```python
from build123d import *

# Parameters (mm, degrees)
F1_DEPTH = 8
F2_R     = 2.5
F3_R     = 5
F4_DEPTH = 5
F5_R     = 5
F6_DEPTH = 5


# Not quite as in the source:
# - a feature names something its author has since deleted; it is built from what else it names


with BuildPart() as f1:
    # F0 (on Front) → F1 (new body)
    with BuildSketch(Plane.XZ):
        with BuildLine():
            ThreePointArc((0, -7.5), (-7.5, 0), (0, 7.5))
            Line((0, 7.5), (-100, 7.5))
            Line((-100, 7.5), (-100, -7.5))
            Line((-100, -7.5), (0, -7.5))
        make_face()
        with BuildLine():
            Line((0, 5), (0, 7.5))
            ThreePointArc((0, 7.5), (-7.5, 0), (0, -7.5))
            Line((0, -7.5), (0, -5))
            ThreePointArc((0, -5), (-5, 0), (0, 5))
        make_face()
        with BuildLine():
            ThreePointArc((0, -7.5), (5.3033008589, -5.3033008589), (7.5, 0))
            ThreePointArc((7.5, 0), (5.3033008589, 5.3033008589), (0, 7.5))
            Line((0, 7.5), (0, 5))
            ThreePointArc((0, 5), (3.5355339059, 3.5355339059), (5, 0))
            ThreePointArc((5, 0), (3.5355339059, -3.5355339059), (0, -5))
            Line((0, -5), (0, -7.5))
        make_face()
    extrude(amount=F1_DEPTH)

    # F2
    f2_edges = [f1.edges().sort_by_distance(p)[0] for p in [
        (-100, -4, 7.5),
        (-100, -4, -7.5),
    ]]
    fillet(f2_edges, radius=F2_R)

    # F3 (on face) → F4 (join)
    with BuildSketch(Plane(origin=(0, 0, 0), x_dir=(-1, 0, 0), z_dir=(0, 1, 0))):
        with Locations((92.5, 0)):
            Circle(F3_R)
    extrude(amount=F4_DEPTH)

    # F5 (on face) → F6 (cut)
    with BuildSketch(Plane.XZ.offset(8)):
        with Locations((-92.5, 0)):
            Circle(F5_R)
    extrude(amount=-F6_DEPTH, mode=Mode.SUBTRACT)


solid = f1.part
```
The model under review builds one solid part; all positions refer to its coordinate system, in mm. A direction names the side the tool comes from. Give positions to 0.01 mm unless a question says otherwise; leave off trailing zeros. Loops run counter-clockwise (first coordinate to the right, second up) from the corner with the lowest first, then second, coordinate; pieces in that order, holes last. Notation, with made-up numbers: (6, 64) -> (21, 64) arc R30 ccw to (21, 94) -> close; hole circle Ø9 at (16, -20.5). An arc over 180 degrees is marked (long way). Use CSV: the item, a comma, the result in double quotes.
1. For P1, Ø5, axis at x = -91.5, z = 0.5, coming from the -Y side; P2, Ø6, axis at y = -6.5, z = 3.5, coming from the +X side; P3, Ø5, axis at y = 0, z = -5, coming from the +X side; P4, Ø6, axis at x = -25, y = 2.5, coming from the +Z side, all flat-tipped, find the tip position at first contact; note any pin that passes through.
Result:
P1,"stops at y = -3"
P2,"stops at x = 7.48"
P3,"stops at x = 7.07"
P4,"stops at z = 7.5"
2. Machinability: for faces 1 (the face through (-99, -4, -7)), 2 (the face through (-93, -3, 0)), which of the approach directions +Z, -Z, +X, -X, +Y, -Y give a long, thin tool a straight path to every point of the face, cutting with its end or side? Answer none if there is none.
Result:
face 1,"-Z, -X, +Y, -Y"
face 2,"-Y"
3. Consider section A-A, the plane z = 4. Write out the cut boundary in (x, y), then the cut area to 3 significant figures.
Result:
outline,"(-100, -8) -> (-95.5, -8) -> (-95.5, -3) -> (-89.5, -3) -> (-89.5, -8) -> (-3, -8) -> (-3, 0) -> (-89.5, 0) -> (-89.5, 5) -> (-95.5, 5) -> (-95.5, 0) -> (-100, 0) -> close; (3, -8) -> (6.34, -8) -> (6.34, 0) -> (3, 0) -> close"
area,"803 mm²"
4. The part is to be moulded in two halves that separate along X. For faces 3 (the face through (-87.881, -5.535, -1.915)), 4 (the face through (-97.119, 2.465, -1.915)), 5 (the face through (-48, -4, 7.5)), 6 (the face through (-100, -4, 0)), say which applies: +X half, -X half, draft (parallel to the pull), parting line (faces both ways), or undercut.
Result:
face 3,"undercut"
face 4,"parting line"
face 5,"draft"
face 6,"-X half"
5. Consider section C-C, the plane z = -2.75. Write out the cut boundary in (x, y), then the cut area to 3 significant figures.
Result:
outline,"(-100, -8) -> (-96.68, -8) -> (-96.68, -3) -> (-88.32, -3) -> (-88.32, -8) -> (-4.18, -8) -> (-4.18, 0) -> (-88.32, 0) -> (-88.32, 5) -> (-96.68, 5) -> (-96.68, 0) -> (-100, 0) -> close; (4.18, -8) -> (6.98, -8) -> (6.98, 0) -> (4.18, 0) -> close"
area,"789 mm²"
6. To check wall thickness, follow probe 1 along Z at (x, y) = (-92.5, -6.75); probe 2 along X at (y, z) = (-5.75, 1); probe 3 along Y at (x, z) = (-88, 0). State the ranges of each line that lie inside material, in increasing order. Write a range as from..to.
Result:
probe 1,"z = -7.5..-5, 5..7.5"
probe 2,"x = -100..-97.4, -87.6..-4.9, 4.9..7.43"
probe 3,"y = -3..5"
7. Consider section B-B, the plane x = -92.5. Write out the cut boundary in (y, z).
Result:
outline,"(-8, -7.5) -> (0, -7.5) -> (0, -5) -> (5, -5) -> (5, 5) -> (0, 5) -> (0, 7.5) -> (-8, 7.5) -> (-8, 5) -> (-3, 5) -> (-3, -5) -> (-8, -5) -> close"
8. Consider section D-D, the plane y = 3.75. Write out the cut boundary in (x, z), then the cut area to 3 significant figures.
Result:
outline,"circle Ø10 at (-92.5, 0)"
area,"78.5 mm²"
